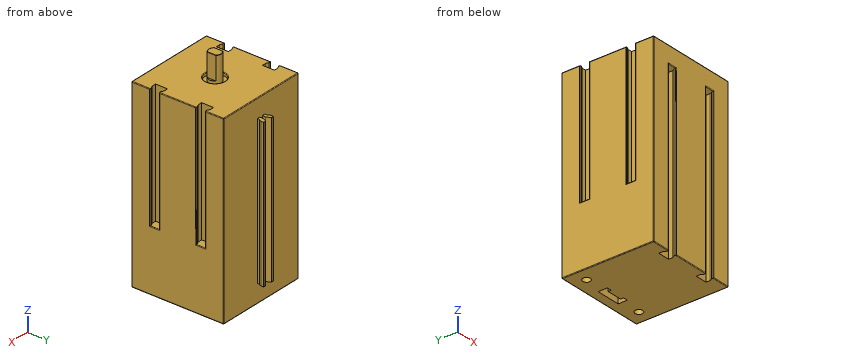
from build123d import *

# Parameters (mm, degrees)
SKETCH_1_W          = 30
SKETCH_1_H          = 30
EXTRUDE_1_DEPTH     = 60
CUT_EXTRUDE_1_DEPTH = 54.5
CUT_EXTRUDE_START   = -60
CUT_EXTRUDE_2_DEPTH = 40
EXTRUDE_START       = -6
EXTRUDE_2_DEPTH     = 48
FILLET_1_R          = 0.1
SKETCH_6_R          = 3.25
CUT_EXTRUDE_3_DEPTH = 1
SKETCH_7_R          = 2
EXTRUDE_3_DEPTH     = 8.5
CUT_EXTRUDE_START_2 = -7.5
CUT_EXTRUDE_5_DEPTH = 7.5
SKETCH_10_R         = 1.25
CUT_EXTRUDE_6_DEPTH = 5
CUT_EXTRUDE_7_DEPTH = 5
FILLET_2_R          = 0.2
FILLET_3_R          = 0.1


with BuildPart() as part:
    # 草图1 → 凸台-拉伸1 (new body)
    with BuildSketch(Plane.XY):
        with Locations((0, 15)):
            Rectangle(SKETCH_1_W, SKETCH_1_H)
    extrude(amount=-EXTRUDE_1_DEPTH)

    # 草图2 → 切除-拉伸1 (cut)
    with BuildSketch(Plane(origin=(0, 0, -60), x_dir=(-1, 0, 0), z_dir=(0, 0, -1))):
        with BuildLine():
            Line((-9, 0.677124344), (-9, 0))
            Line((-9, 0), (-6, 0))
            Line((-6, 0), (-6, 0.677124344))
            ThreePointArc((-6, 0.677124344), (-5.719957697, 1.088161527), (-5.55, 1.555590279))
            Line((-5.55, 1.555590279), (-5.55, 2.8))
            Line((-5.55, 2.8), (-9.45, 2.8))
            Line((-9.45, 2.8), (-9.45, 1.555590279))
            ThreePointArc((-9.45, 1.555590279), (-9.280042303, 1.088161527), (-9, 0.677124344))
        make_face()
        with BuildLine():
            Line((5.55, 2.8), (5.55, 1.555590279))
            ThreePointArc((5.55, 1.555590279), (5.719957697, 1.088161527), (6, 0.677124344))
            Line((6, 0.677124344), (6, 0))
            Line((6, 0), (9, 0))
            Line((9, 0), (9, 0.677124344))
            ThreePointArc((9, 0.677124344), (9.280042303, 1.088161527), (9.45, 1.555590279))
            Line((9.45, 1.555590279), (9.45, 2.8))
            Line((9.45, 2.8), (5.55, 2.8))
        make_face()
    extrude(amount=-CUT_EXTRUDE_1_DEPTH, mode=Mode.SUBTRACT)

    # 草图3 → 切除-拉伸2 (cut)
    with BuildSketch(Plane(origin=(0, 0, -60), x_dir=(-1, 0, 0), z_dir=(0, 0, -1)).offset(CUT_EXTRUDE_START)):
        with BuildLine():
            Line((-14.322875656, 9), (-15, 9))
            Line((-15, 9), (-15, 6))
            Line((-15, 6), (-14.322875656, 6))
            ThreePointArc((-14.322875656, 6), (-13.911838473, 5.719957697), (-13.444409721, 5.55))
            Line((-13.444409721, 5.55), (-12.2, 5.55))
            Line((-12.2, 5.55), (-12.2, 9.45))
            Line((-12.2, 9.45), (-13.444409721, 9.45))
            ThreePointArc((-13.444409721, 9.45), (-13.911838473, 9.280042303), (-14.322875656, 9))
        make_face()
        with BuildLine():
            Line((-12.2, 20.55), (-13.444409721, 20.55))
            ThreePointArc((-13.444409721, 20.55), (-13.911838473, 20.719957697), (-14.322875656, 21))
            Line((-14.322875656, 21), (-15, 21))
            Line((-15, 21), (-15, 24))
            Line((-15, 24), (-14.322875656, 24))
            ThreePointArc((-14.322875656, 24), (-13.911838473, 24.280042303), (-13.444409721, 24.45))
            Line((-13.444409721, 24.45), (-12.2, 24.45))
            Line((-12.2, 24.45), (-12.2, 20.55))
        make_face()
        with BuildLine():
            Line((14.322875656, 21), (15, 21))
            Line((15, 21), (15, 24))
            Line((15, 24), (14.322875656, 24))
            ThreePointArc((14.322875656, 24), (13.911838473, 24.280042303), (13.444409721, 24.45))
            Line((13.444409721, 24.45), (12.2, 24.45))
            Line((12.2, 24.45), (12.2, 20.55))
            Line((12.2, 20.55), (13.444409721, 20.55))
            ThreePointArc((13.444409721, 20.55), (13.911838473, 20.719957697), (14.322875656, 21))
        make_face()
        with BuildLine():
            Line((12.2, 9.45), (13.444409721, 9.45))
            ThreePointArc((13.444409721, 9.45), (13.911838473, 9.280042303), (14.322875656, 9))
            Line((14.322875656, 9), (15, 9))
            Line((15, 9), (15, 6))
            Line((15, 6), (14.322875656, 6))
            ThreePointArc((14.322875656, 6), (13.911838473, 5.719957697), (13.444409721, 5.55))
            Line((13.444409721, 5.55), (12.2, 5.55))
            Line((12.2, 5.55), (12.2, 9.45))
        make_face()
    extrude(amount=CUT_EXTRUDE_2_DEPTH, mode=Mode.SUBTRACT)

    # 草图5 → 凸台-拉伸2 (add)
    with BuildSketch(Plane(origin=(0, 0, -60), x_dir=(-1, 0, 0), z_dir=(0, 0, -1)).offset(EXTRUDE_START)):
        with BuildLine():
            Line((-1.5, 30.677124344), (-1.5, 30))
            Line((-1.5, 30), (-0.5, 30))
            Line((-0.5, 30), (-0.5, 31.07225346))
            Line((-0.5, 31.07225346), (-1.165769145, 32.5))
            Line((-1.165769145, 32.5), (-1.95, 32.5))
            Line((-1.95, 32.5), (-1.95, 31.555590279))
            ThreePointArc((-1.95, 31.555590279), (-1.780042303, 31.088161527), (-1.5, 30.677124344))
        make_face()
        with BuildLine():
            Line((1.5, 30), (1.5, 30.677124344))
            ThreePointArc((1.5, 30.677124344), (1.780042303, 31.088161527), (1.95, 31.555590279))
            Line((1.95, 31.555590279), (1.95, 32.5))
            Line((1.95, 32.5), (1.165769145, 32.5))
            Line((1.165769145, 32.5), (0.5, 31.07225346))
            Line((0.5, 31.07225346), (0.5, 30))
            Line((0.5, 30), (1.5, 30))
        make_face()
    extrude(amount=-EXTRUDE_2_DEPTH)

    # 圆角1
    fillet_1_edges = [part.edges().sort_by_distance(p)[0] for p in [
        (1.557884573, 32.5, -6),
        (1.95, 32.5, -30),
        (1.165769145, 32.5, -30),
        (1.557884573, 32.5, -54),
        (-1.557884573, 32.5, -6),
        (-1.165769145, 32.5, -30),
        (-1.95, 32.5, -30),
        (-1.557884573, 32.5, -54),
    ]]
    fillet(fillet_1_edges, radius=FILLET_1_R)

    # 草图6 → 切除-拉伸3 (cut)
    with BuildSketch(Plane.XY):
        with Locations((0, 15)):
            Circle(SKETCH_6_R)
    extrude(amount=-CUT_EXTRUDE_3_DEPTH, mode=Mode.SUBTRACT)

    # 草图7 → 凸台-拉伸3 (add)
    with BuildSketch(Plane.XY.offset(-1)):
        with Locations((0, 15)):
            Circle(SKETCH_7_R)
    extrude(amount=EXTRUDE_3_DEPTH)

    # 草图9 → 切除-拉伸5 (cut)
    with BuildSketch(Plane.XY.offset(7.5).offset(CUT_EXTRUDE_START_2)):
        with BuildLine():
            Line((-1.4, 16.428285686), (-1.4, 13.571714314))
            ThreePointArc((-1.4, 13.571714314), (-2, 15), (-1.4, 16.428285686))
        make_face()
        with BuildLine():
            Line((1.4, 16.428285686), (1.4, 13.571714314))
            ThreePointArc((1.4, 13.571714314), (2, 15), (1.4, 16.428285686))
        make_face()
    extrude(amount=CUT_EXTRUDE_5_DEPTH, mode=Mode.SUBTRACT)

    # 草图10 → 切除-拉伸6 (cut)
    with BuildSketch(Plane(origin=(0, 0, -60), x_dir=(-1, 0, 0), z_dir=(0, 0, -1))):
        with Locations((-10.5, 25.5)):
            Circle(SKETCH_10_R)
        with Locations((10.5, 25.5)):
            Circle(SKETCH_10_R)
    extrude(amount=-CUT_EXTRUDE_6_DEPTH, mode=Mode.SUBTRACT)

    # 草图11 → 切除-拉伸7 (cut)
    with BuildSketch(Plane(origin=(0, 0, -60), x_dir=(-1, 0, 0), z_dir=(0, 0, -1))):
        Polygon((2.5, 24), (4, 24), (4, 27), (-4, 27), (-4, 24), (-2.5, 24), (-2.5, 25), (2.5, 25), align=None)
    extrude(amount=-CUT_EXTRUDE_7_DEPTH, mode=Mode.SUBTRACT)

    # 圆角2
    fillet_2_edges = [part.edges().sort_by_distance(p)[0] for p in [
        (15, 15, -60),
        (-15, 15, 0),
        (-15, 21, -20),
        (-15, 24, -20),
        (-15, 22.5, -40),
        (-15, 3, 0),
        (0, 30, -60),
        (-15, 6, -20),
        (-15, 9, -20),
        (-15, 7.5, -40),
        (12, 0, -60),
        (7.5, 0, -5.5),
        (6, 0, -32.75),
        (9, 0, -32.75),
        (-3.25, 15, 0),
        (0, 0, -60),
        (-15, 15, -60),
        (-7.5, 0, -5.5),
        (-9, 0, -32.75),
        (-6, 0, -32.75),
        (0, 30, 0),
        (15, 3, 0),
        (0, 0, 0),
        (-15, 27, 0),
        (15, 15, 0),
        (15, 9, -20),
        (15, 6, -20),
        (-12, 0, -60),
        (15, 7.5, -40),
        (-15, 30, -30),
        (15, 30, -30),
        (15, 0, -30),
        (-15, 0, -30),
        (15, 27, 0),
        (15, 24, -20),
        (15, 21, -20),
        (15, 22.5, -40),
    ]]
    fillet(fillet_2_edges, radius=FILLET_2_R)

    # 圆角3
    fillet_3_edges = [part.edges().sort_by_distance(p)[0] for p in [
        (0, 17, 7.5),
        (1.4, 15, 7.5),
        (0, 13, 7.5),
        (-1.4, 15, 7.5),
    ]]
    fillet(fillet_3_edges, radius=FILLET_3_R)


solid = part.part
CAD build for the part. Positions are in the model's coordinates, mm. Give positions to 0.01 mm unless a question says otherwise; leave off trailing zeros. Loops run counter-clockwise (first coordinate to the right, second up) from the corner with the lowest first, then second, coordinate; pieces in that order, holes last. Notation, with made-up numbers: M 81.5,54 L 102.5,54 A31 cw 102.5,86 Z; hole C 62,0 d10. An arc over 180 degrees is marked long. Answer in a Markdown table with one row per item. Add a question column.
Item 1: Band-saw the part on D-D on y = 15. Give the cut face in (x, z).
Item 2: Drop flat-ended pins along their axis: P1, Ø10, axis at y = 21.5, z = -29, coming from the +X side; P2, Ø1, axis at x = -0.5, z = -28.5, coming from the +Y side; P3, Ø0.7, axis at x = -1, y = 31, coming from the -Z side; P4, Ø0.9, axis at y = 30.5, z = -36.5, coming from the -X side. Give the stop position or say it passes through.
Item 3: Band-saw the part on C-C on x = 10.5. Give the cut face in (y, z), then the cut area to 3 significant figures.
Item 4: Probe probe 1 along Y at (x, z) = (0, -0.8); probe 2 along Y at (x, z) = (-13, -34); probe 3 along X at (y, z) = (2, -44.5). List the from-to ranges inside material, lowest first.
Item 5: Band-saw the part on A-A on y = 4. Give the cut face in (x, z), then the cut area to 3 significant figures.
Item 6: Band-saw the part on B-B on x = 7. Give the cut face in (y, z).
Reply:
| question | item | result |
|---|---|---|
| 1 | outline | M -15,-59.8 A0.2 ccw -14.8,-60 L 14.8,-60 A0.2 ccw 15,-59.8 L 15,-0.2 A0.2 ccw 14.8,0 L 3.45,0 A0.2 ccw 3.25,-0.2 L 3.25,-1 L 2,-1 L 2,0 L 1.4,0 L 1.4,7.4 A0.1 ccw 1.3,7.5 L -1.3,7.5 A0.1 ccw -1.4,7.4 L -1.4,0 L -2,0 L -2,-1 L -3.25,-1 L -3.25,-0.2 A0.2 ccw -3.45,0 L -14.8,0 A0.2 ccw -15,-0.2 Z |
| 2 | P1 | stops at x = 15 |
| 2 | P2 | stops at y = 32.14 |
| 2 | P3 | stops at z = -54 |
| 2 | P4 | stops at x = -1.7 |
| 3 | outline | M 0,-59.8 A0.2 ccw 0.2,-60 L 24.25,-60 L 24.25,-55 L 26.75,-55 L 26.75,-60 L 29.8,-60 A0.2 ccw 30,-59.8 L 30,-0.2 A0.2 ccw 29.8,0 L 0.2,0 A0.2 ccw 0,-0.2 Z |
| 3 | area | 1,790 mm^2 |
| 4 | probe 1 | y = 0 to 11.75, 13 to 17, 18.25 to 30 |
| 4 | probe 2 | y = 0 to 5.55, 9.45 to 20.55, 24.45 to 30 |
| 4 | probe 3 | x = -15 to -9.45, -5.55 to 5.55, 9.45 to 15 |
| 5 | outline | M -15,-59.8 A0.2 ccw -14.8,-60 L 14.8,-60 A0.2 ccw 15,-59.8 L 15,-0.2 A0.2 ccw 14.8,0 L -14.8,0 A0.2 ccw -15,-0.2 Z |
| 5 | area | 1,800 mm^2 |
| 6 | outline | M 0,-5.3 A0.2 ccw 0.2,-5.5 L 2.8,-5.5 L 2.8,-60 L 29.8,-60 A0.2 ccw 30,-59.8 L 30,-0.2 A0.2 ccw 29.8,0 L 0.2,0 A0.2 ccw 0,-0.2 Z |
